Check sheet for the drawn part. Datum: minimum x, y, z corner. Units: mm. Give positions to 0.01 mm unless a question says otherwise; leave off trailing zeros. Loops run counter-clockwise (first coordinate to the right, second up) from the corner with the lowest first, then second, coordinate; pieces in that order, holes last. Notation, with made-up numbers: (-14, -16) - (-7, -16) arc R25 cw to (-7, 15) - close; hole circle Ø11 at (-18, 77.5). An arc over 180 degrees is marked (long way). Use a Markdown table: item, result. Add a question column.
1. Cross-section at C-C on x = 28. Enter the section's corners in (y, z), and give its area (3 significant figures).
2. Material ranges on L1, parallel to X at y = 30, z = 1.85; L2, parallel to X at y = 30.5, z = 1.4 (1 decimal); L3, parallel to X at y = 53.5, z = 1.9, recorded low to high.
3. Depth check by flat-ended pin: P1, Ø1, axis at x = 40, z = 0.5, coming from the -Y side. Enter the tip coordinate at first touch or a pass-through.
4. Cross-section at B-B on x = 7.5. Enter the section's corners in (y, z).
5. Cross-section at D-D on z = 2. Enter the section's corners in (x, y), and give its area (3 significant figures).
6. Cross-section at A-A on y = 30. Enter the section's corners in (x, z).
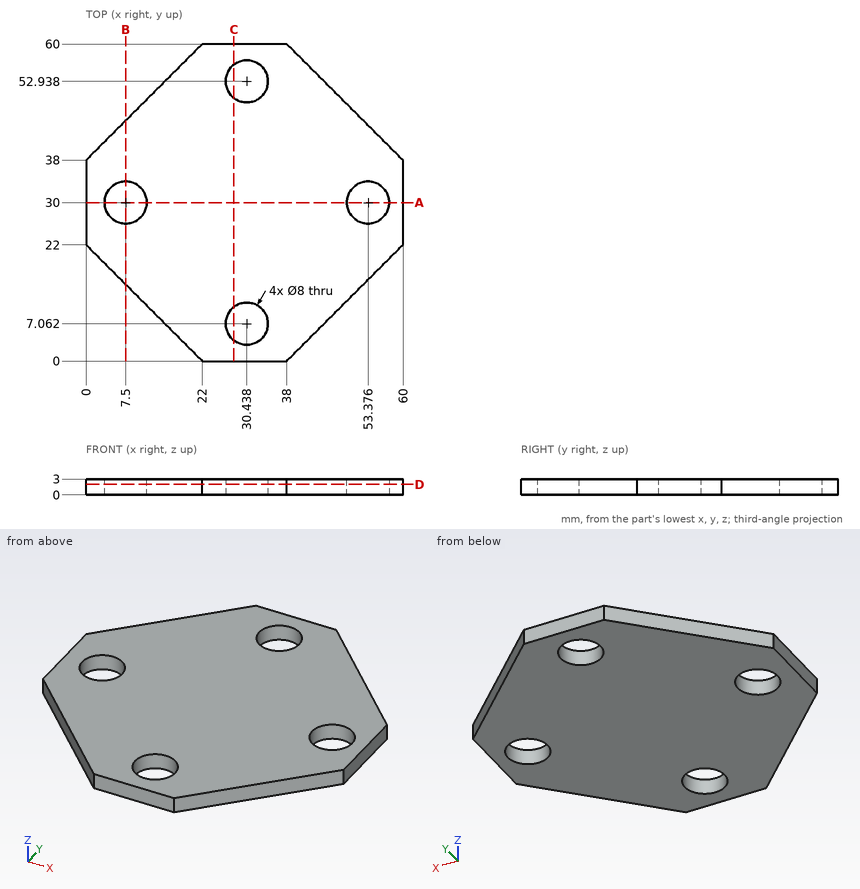
Values found:
| question | item | result |
|---|---|---|
| 1 | outline | (0, 0) - (3.89, 0) - (3.89, 3) - (0, 3) - close; (10.23, 0) - (49.77, 0) - (49.77, 3) - (10.23, 3) - close; (56.11, 0) - (60, 0) - (60, 3) - (56.11, 3) - close |
| 1 | area | 142 mm2 |
| 2 | L1 | x = 0 to 3.5, 11.5 to 49.38, 57.38 to 60 |
| 2 | L2 | x = 0 to 3.5, 11.5 to 49.4, 57.3 to 60 |
| 2 | L3 | x = 15.5 to 26.48, 34.4 to 44.5 |
| 3 | P1 | stops at y = 1.5 |
| 4 | outline | (14.5, 0) - (26, 0) - (26, 3) - (14.5, 3) - close; (34, 0) - (45.5, 0) - (45.5, 3) - (34, 3) - close |
| 5 | outline | (0, 22) - (22, 0) - (38, 0) - (60, 22) - (60, 38) - (38, 60) - (22, 60) - (0, 38) - close; hole circle Ø8 at (7.5, 30); hole circle Ø8 at (30.44, 7.06); hole circle Ø8 at (30.44, 52.94); hole circle Ø8 at (53.38, 30) |
| 5 | area | 2,430 mm2 |
| 6 | outline | (0, 0) - (3.5, 0) - (3.5, 3) - (0, 3) - close; (11.5, 0) - (49.38, 0) - (49.38, 3) - (11.5, 3) - close; (57.38, 0) - (60, 0) - (60, 3) - (57.38, 3) - close |
